from build123d import *

# Parameters (mm, degrees)
SKETCH_R           = 28
SKETCH_R_2         = 7
PAD_DEPTH          = 6
SKETCH007_R        = 12
SKETCH007_R_2      = 8.6
POCKET002_DEPTH    = 2
SKETCH001_R        = 4
PAD001_DEPTH       = 3
PAD002_DEPTH       = 3.5
POLARPATTERN_COUNT = 3
SKETCH003_R        = 1.7
SKETCH003_R_2      = 1.5
POCKET001_DEPTH    = 3.5
POCKET_DEPTH       = 3.4
CHAMFER_SIZE       = 1
CHAMFER001_SIZE    = 1
CHAMFER002_SIZE    = 1
SKETCH008_R        = 8.6
POCKET003_DEPTH    = 2.5


with BuildPart() as part:
    # Sketch → Pad (new body)
    with BuildSketch(Plane.XY.offset(25)):
        Circle(SKETCH_R)
        Circle(SKETCH_R_2, mode=Mode.SUBTRACT)
    extrude(amount=PAD_DEPTH)

    # Sketch007 → Pocket002 (cut)
    with BuildSketch(Plane.XY.offset(31)):
        with Locations((0, 22.5)):
            Circle(SKETCH007_R)
        with Locations((-19.485572, -11.25)):
            Circle(SKETCH007_R)
        with Locations((19.485572, -11.25)):
            Circle(SKETCH007_R)
        Circle(SKETCH007_R_2)
    extrude(amount=-POCKET002_DEPTH, mode=Mode.SUBTRACT)

    # Sketch001 → Pad001 (new body)
    with BuildSketch(Plane.XY.offset(29)):
        with Locations((0, 22.5)):
            Circle(SKETCH001_R)
        with Locations((-19.485572, -11.25)):
            Circle(SKETCH001_R)
        with Locations((19.485572, -11.25)):
            Circle(SKETCH001_R)
    extrude(amount=PAD001_DEPTH)

    # Sketch005 → Pad002 (new body)
    with BuildSketch(Plane.XY.offset(31)):
        with BuildLine():
            Line((-2.25, -8.300452), (-2.25, -17.858821))
            ThreePointArc((-2.25, -17.858821), (0, -18), (2.25, -17.858821))
            Line((2.25, -8.300452), (2.25, -17.858821))
            ThreePointArc((-2.25, -8.300452), (0, -8.6), (2.25, -8.300452))
        make_face()
    pad002 = extrude(amount=PAD002_DEPTH)

    # PolarPattern: Pad002 ×3 about axis
    polarpattern_axis = Axis((0, 0, 31), (0, 0, 1))
    for i in range(1, POLARPATTERN_COUNT):
        add(pad002.rotate(polarpattern_axis, i * 360 / POLARPATTERN_COUNT))

    # Sketch003 → Pocket001 (cut)
    with BuildSketch(Plane.XY.offset(32)):
        with Locations((0, 22.5)):
            Circle(SKETCH003_R)
        with Locations((-19.485572, -11.25)):
            Circle(SKETCH003_R)
        with Locations((19.485572, -11.25)):
            Circle(SKETCH003_R)
        with Locations((-19.485572, 11.25)):
            Circle(SKETCH003_R_2)
        with Locations((19.485572, 11.25)):
            Circle(SKETCH003_R_2)
        with Locations((0, -22.5)):
            Circle(SKETCH003_R_2)
    extrude(amount=-POCKET001_DEPTH, mode=Mode.SUBTRACT)

    # Sketch004 → Pocket (cut)
    with BuildSketch(Plane(origin=(0, 0, 25), x_dir=(1, 0, 0), z_dir=(0, 0, -1))):
        Polygon((-16.685572, 9.633419), (-16.685572, 12.866581), (-19.485572, 14.483162), (-22.285572, 12.866581), (-22.285572, 9.633419), (-19.485572, 8.016838), align=None)
        Polygon((-2.8, 24.116581), (-2.8, 20.883419), (0, 19.266838), (2.8, 20.883419), (2.8, 24.116581), (0, 25.733162), align=None)
        Polygon((19.485572, 14.483162), (16.685572, 12.866581), (16.685572, 9.633419), (19.485572, 8.016838), (22.285572, 9.633419), (22.285572, 12.866581), align=None)
        Polygon((19.485572, -8.016838), (16.685572, -9.633419), (16.685572, -12.866581), (19.485572, -14.483162), (22.285572, -12.866581), (22.285572, -9.633419), align=None)
        Polygon((-22.285572, -9.633419), (-22.285572, -12.866581), (-19.485572, -14.483162), (-16.685572, -12.866581), (-16.685572, -9.633419), (-19.485572, -8.016838), align=None)
        Polygon((-2.8, -20.883419), (-2.8, -24.116581), (0, -25.733162), (2.8, -24.116581), (2.8, -20.883419), (0, -19.266838), align=None)
    extrude(amount=-POCKET_DEPTH, mode=Mode.SUBTRACT)

    # Chamfer
    chamfer_edges = [part.edges().sort_by_distance(p)[0] for p in [
        (15.485572, -11.25, 32),
    ]]
    chamfer(chamfer_edges, length=CHAMFER_SIZE)

    # Chamfer001
    chamfer001_edges = [part.edges().sort_by_distance(p)[0] for p in [
        (-23.485572, -11.25, 32),
    ]]
    chamfer(chamfer001_edges, length=CHAMFER001_SIZE)

    # Chamfer002
    chamfer002_edges = [part.edges().sort_by_distance(p)[0] for p in [
        (-4, 22.5, 32),
    ]]
    chamfer(chamfer002_edges, length=CHAMFER002_SIZE)

    # Sketch008 → Pocket003 (cut)
    with BuildSketch(Plane.XY.offset(31)):
        Circle(SKETCH008_R)
    extrude(amount=-POCKET003_DEPTH, mode=Mode.SUBTRACT)


solid = part.part
Can you work these out from the model? Positions are in its coordinate system, mm. A direction names the side the tool comes from. Give positions to 0.01 mm unless a question says otherwise; leave off trailing zeros. Order: outer loops, then holes, each group sorted by start corner. A loop starts at its lowest first (then second) coordinate and runs counter-clockwise, first axis right, second up. Notation, with made-up numbers: M 13.25,2 L 43.25,2 A30 ccw 43.25,36 Z; hole C -18.75,-25.5 d7. An arc over 180 degrees is marked long. Use a Markdown table: item, result. Add a question column.
Item 1: For faces 4 (the flat face through (-16.686, -11, 27)), 5 (the flat face through (0, 20.5, 32)), 6 (the flat face through (0, 17, 29)), which set-ups out of +Z, -Z, +X, -X, +Y, -Y let a thin tool reach every point of the face, with its end or its side?
Item 2: Suppose I cut it at A-A (z = 32.75). List the corners of the cut face in (x, y) for me, then the cut area to 3 significant figures.
Item 3: Suppose I cut it at D-D (y = -16.5). List the corners of the cut face in (x, z) for me.
Item 4: Suppose I cut it at C-C (x = -10). List the corners of the cut face in (y, z) for me, then the cut area to 3 significant figures.
Item 5: Suppose I cut it at B-B (y = 22.5). List the corners of the cut face in (x, z) for me.
Item 6: Will these pins go through, and if not, where does the flat tip stop? pin 1 (1.8 mm diameter, centred on y = -12, z = 33.5, fed in from +X); pin 2 (3 mm diameter, centred on x = 16.5, y = -19.5, fed in from +Z); pin 3 (4 mm diameter, centred on y = 6.5, z = 28.5, fed in from -X); pin 4 (8 mm diameter, centred on x = -1, y = -21.5, fed in from +Z).
Item 7: We'd pull the mould along Y, two halves only. Please class faces 1 (the flat face through (-20.866, 8.814, 26.676)), 2 (the flat face through (21, -13, 32)), 3 (the flat face through (22.286, 11, 27)): +Y half, -Y half, draft (parallel to the pull), parting line (faces both ways), or undercut.
Item 8: If I drill on L1, parallel to Y at x = 0, z = 27.55; L2, parallel to Y at x = 0, z = 29.65; L3, parallel to Y at x = 22, z = 26.25, over which ranges is the centre line in solid material (lowest first)? Write a range as [from, to].
Answer sheet:
| question | item | result |
|---|---|---|
| 1 | face 4 | -Z |
| 1 | face 5 | +Z, +X, -X, +Y |
| 1 | face 6 | +Z |
| 2 | outline | M -16.59,6.98 L -8.31,2.2 A8.6 cw -6.06,6.1 L -14.34,10.88 A18 ccw Z; M -2.25,-17.86 A18 ccw 2.25,-17.86 L 2.25,-8.3 A8.6 cw -2.25,-8.3 Z; M 6.06,6.1 A8.6 cw 8.31,2.2 L 16.59,6.98 A18 ccw 14.34,10.88 Z |
| 2 | area | 128 mm² |
| 3 | outline | M -22.62,25 L 22.62,25 L 22.62,29 L 8.69,29 L 8.69,31 L 2.25,31 L 2.25,34.5 L -2.25,34.5 L -2.25,31 L -8.69,31 L -8.69,29 L -22.62,29 Z |
| 4 | outline | M -26.15,25 L 26.15,25 L 26.15,29 L 15.87,29 L 15.87,31 L 8.37,31 L 8.37,34.5 L 3.18,34.5 L 3.18,31 L -3.9,31 L -3.9,29 L -18.6,29 L -18.6,31 L -26.15,31 Z |
| 4 | area | 282 mm² |
| 5 | outline | M -16.67,25 L -2.8,25 L -2.8,28.4 L 2.8,28.4 L 2.8,25 L 16.67,25 L 16.67,31 L 12,31 L 12,29 L 4,29 L 4,31 L 3,32 L 1.7,32 L 1.7,28.5 L -1.7,28.5 L -1.7,32 L -3,32 L -4,31 L -4,29 L -12,29 L -12,31 L -16.67,31 Z |
| 6 | pin 1 | stops at x = 2.25 |
| 6 | pin 2 | stops at z = 29 |
| 6 | pin 3 | stops at x = -27.64 |
| 6 | pin 4 | stops at z = 34.5 |
| 7 | face 1 | undercut |
| 7 | face 2 | draft |
| 7 | face 3 | undercut |
| 8 | L1 | y = [-28, -25.73], [-19.27, -7], [7, 19.27], [25.73, 28] |
| 8 | L2 | y = [-28, -24], [-21, -8.6], [8.6, 10.5], [18.5, 20.8], [24.2, 26.5] |
| 8 | L3 | y = [-17.32, -13.03], [-9.47, 9.47], [13.03, 17.32] |
